Here's the drawing with two shaded views (mm, measured from the low corner). I have some questions. A direction names the side the tool comes from. Give positions to 0.01 mm unless a question says otherwise; leave off trailing zeros. Loops run counter-clockwise (first coordinate to the right, second up) from the corner with the lowest first, then second, coordinate; pieces in that order, holes last. Notation, with made-up numbers: M 53.5,-7 L 63.5,-7 A18 cw 63.5,4 Z; hole C 75,25 d5. An arc over 180 degrees is marked long. Put each result on its own line as item: value. Start each with the question number.
1) If we mould it in two halves opening along X, with no side actions, what happens to the marked faces 1, 2 and 3? For each: +X half, -X half, draft (parallel to the pull), parting line (faces both ways), or undercut.
2) Imagine slicing it at B-B (z = 44.45). Write out the boundary of the cut face in (x, y).
3) For P1, Ø14, axis at x = 124.5, y = 14, coming from the +Z side; P2, Ø6, axis at x = 110.5, z = 16.5, coming from the -Y side; P3, Ø3.5, axis at x = 119, y = 29.5, coming from the +Z side; P4, Ø23, axis at x = 184.912, z = 44.45, coming from the +Y side, each with a flat end and sliding along its axis, tell me the tip position at first contact or that it passes through.
4) Imagine slicing it at A-A (x = 129.54). Write out the boundary of the cut face in (y, z), then the cut area to 3 significant figures.
5) Imagine slicing it at D-D (z = 141.5). Write out the boundary of the cut face in (x, y).
6) Imagine slicing it at C-C (y = 10). Write out the boundary of the cut face in (x, z).
7) For the marked faces 4 and 5, which set-ups out of +Z, -Z, +X, -X, +Y, -Y let a thin tool reach every point of the face, with its end or its side?
8) Please list where these lines run through material, in increasing order: line 1 along X through (y, z) = (29.7, 44.45); line 2 along X through (y, z) = (19, 20.5); line 3 along Z through (x, y) = (185, 14). Write a range as from..to.
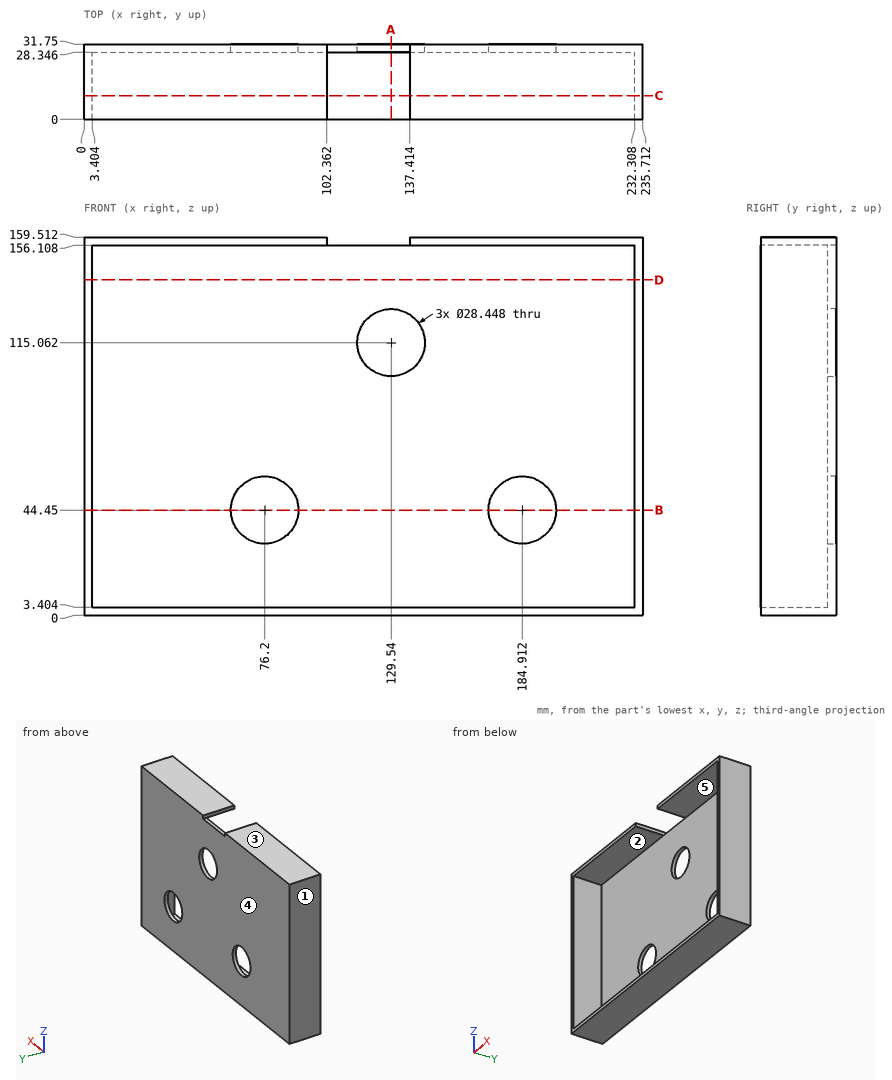
Recorded:
1. face 1: -X half
1. face 2: undercut
1. face 3: draft
2. outline: M 0,0 L 3.4,0 L 3.4,28.35 L 61.98,28.35 L 61.98,31.75 L 0,31.75 Z; M 90.42,28.35 L 170.69,28.35 L 170.69,31.75 L 90.42,31.75 Z; M 199.14,28.35 L 232.31,28.35 L 232.31,0 L 235.71,0 L 235.71,31.75 L 199.14,31.75 Z
3. P1: z = 3.4
3. P2: y = 28.35
3. P3: z = 156.11
3. P4: through
4. outline: M 0,0 L 31.75,0 L 31.75,100.84 L 28.35,100.84 L 28.35,3.4 L 0,3.4 Z; M 28.35,129.29 L 31.75,129.29 L 31.75,156.11 L 28.35,156.11 Z
4. area: 531 mm²
5. outline: M 0,0 L 3.4,0 L 3.4,28.35 L 232.31,28.35 L 232.31,0 L 235.71,0 L 235.71,31.75 L 0,31.75 Z
6. outline: M 0,0 L 235.71,0 L 235.71,159.51 L 137.41,159.51 L 137.41,156.11 L 232.31,156.11 L 232.31,3.4 L 3.4,3.4 L 3.4,156.11 L 102.36,156.11 L 102.36,159.51 L 0,159.51 Z
7. face 4: +Z, -Z, +X, -X, +Y
7. face 5: -Y
8. line 1: 0..61.98, 90.42..170.69, 199.14..235.71
8. line 2: 0..3.4, 232.31..235.71
8. line 3: 0..3.4, 156.11..159.51
